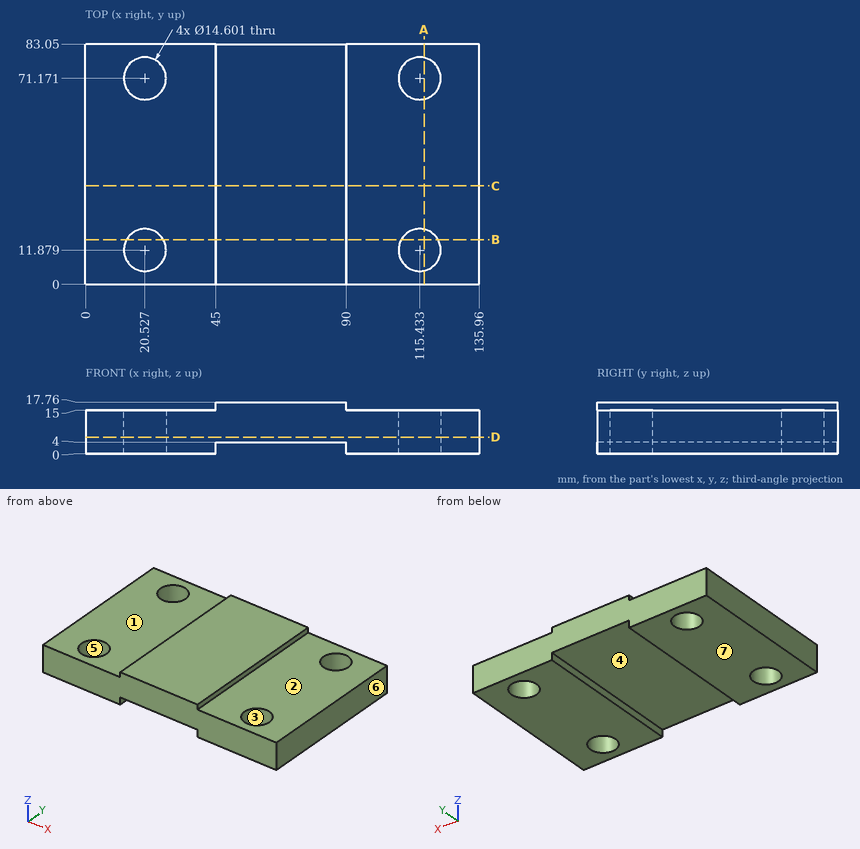
Study the drawing (mm; zero at the part's minimum x, y, z) and answer. A direction names the side the tool comes from. Round coordinates to 2 decimals unless told otherwise and drop trailing zeros. Order: outer loops, then holes, each group sorted by start corner. A loop starts at its lowest first (then second) coordinate and runs counter-clockwise, first axis right, second up. Notation, with made-up numbers: (19, 49) -> (51, 49) arc R23 ccw to (51, 85) -> close; hole circle Ø10 at (43.25, 38.5). An arc over 180 degrees is marked (long way). Answer as CSV lines item,"result". Start each with the question number.
(1) The part is cut by section A-A (x = 117). Determine the outline of the cut face in (y, z), then the cut area to 3 significant figures.
(2) The part is cut by section B-B (y = 15.5). Determine the outline of the cut face in (x, z).
(3) Flat-ended cylindrical pins translate along their axes: pin 1 Ø1.4 at (y, z) = (39, 16.5) entering from +X; pin 2 Ø11.5 at (x, y) = (20.53, 11.88) entering from +Z; pin 3 Ø0.8 at (y, z) = (54, 16.5) entering from -X; pin 4 Ø22.5 at (x, y) = (24, 30.5) entering from +Z. Find the tip coordinate at first contact, or state that the pin passes through.
(4) A tool of negligible diameter and unlimited length cuts with its end or side. For the marked faces 1, 2, 3 and 4, from which of +Z, -Z, +X, -X, +Y, -Y can it reach the whole face along a straight path? Write none if from no direction.
(5) Find the intervals of material crossed by probe 1 along Y at (x, z) = (20, 9.25); probe 2 along X at (y, z) = (39.5, 3.5); probe 3 along X at (y, z) = (73, 9.25) (1 decimal), in increasing order. Write a range as from..to.
(6) The part is cut by section D-D (z = 5.75). Determine the outline of the cut face in (x, y).
(7) For a pull along X with two mould halves and no side action, classify the marked faces 5, 6 and 7 as +X half, -X half, draft (parallel to the pull), parting line (faces both ways), or undercut.
(8) The part is cut by section C-C (y = 34). Determine the outline of the cut face in (x, z).
Evaluation:
1,outline,"(0, 0) -> (4.75, 0) -> (4.75, 15) -> (0, 15) -> close; (19.01, 0) -> (64.04, 0) -> (64.04, 15) -> (19.01, 15) -> close; (78.3, 0) -> (83.05, 0) -> (83.05, 15) -> (78.3, 15) -> close"
1,area,"818 mm²"
2,outline,"(0, 0) -> (14.19, 0) -> (14.19, 15) -> (0, 15) -> close; (26.87, 0) -> (45, 0) -> (45, 4) -> (90, 4) -> (90, 0) -> (109.09, 0) -> (109.09, 15) -> (90, 15) -> (90, 17.76) -> (45, 17.76) -> (45, 15) -> (26.87, 15) -> close; (121.77, 0) -> (135.96, 0) -> (135.96, 15) -> (121.77, 15) -> close"
3,pin 1,"x = 90"
3,pin 2,"through"
3,pin 3,"x = 45"
3,pin 4,"z = 15"
4,face 1,"+Z, -X, +Y, -Y"
4,face 2,"+Z, +X, +Y, -Y"
4,face 3,"+Z, -Z"
4,face 4,"-Z, +Y, -Y"
5,probe 1,"0..4.6, 19.16..63.89, 78.45..83.05"
5,probe 2,"0..45, 90..135.96"
5,probe 3,"0..13.5, 27.6..108.4, 122.5..136"
6,outline,"(0, 0) -> (135.96, 0) -> (135.96, 83.05) -> (0, 83.05) -> close; hole circle Ø14.6 at (20.53, 11.88); hole circle Ø14.6 at (20.53, 71.17); hole circle Ø14.6 at (115.43, 11.88); hole circle Ø14.6 at (115.43, 71.17)"
7,face 5,"undercut"
7,face 6,"+X half"
7,face 7,"draft"
8,outline,"(0, 0) -> (45, 0) -> (45, 4) -> (90, 4) -> (90, 0) -> (135.96, 0) -> (135.96, 15) -> (90, 15) -> (90, 17.76) -> (45, 17.76) -> (45, 15) -> (0, 15) -> close"
